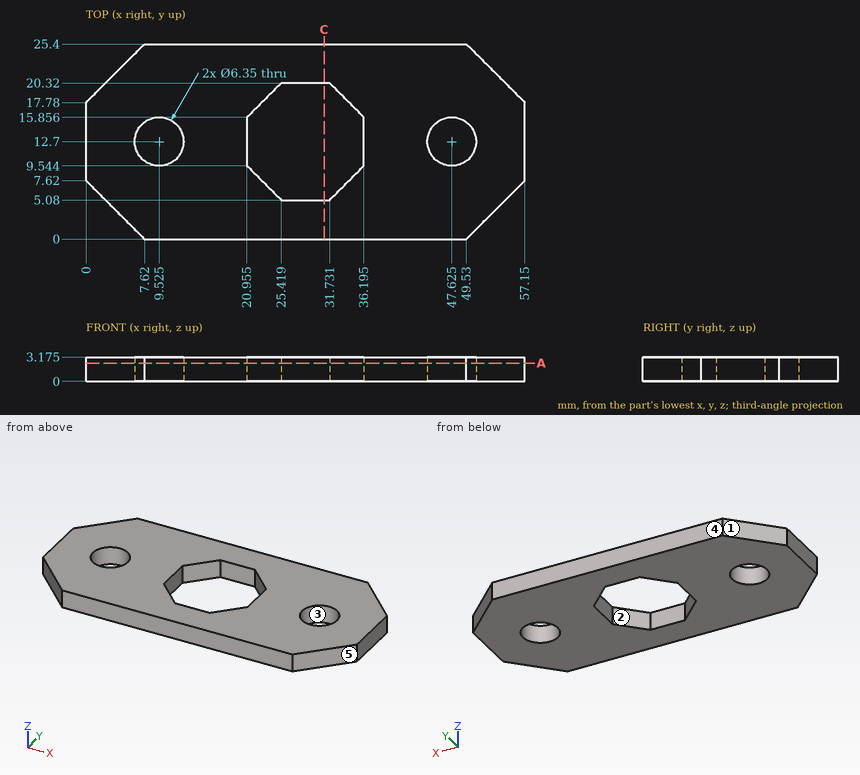
Geometry check sheet. Reference: drawing and pictorial views, mm from the part's lowest x, y, z. A direction names the side the tool comes from. Round coordinates to 2 decimals unless told otherwise and drop trailing zeros. Loops run counter-clockwise (first coordinate to the right, second up) from the corner with the lowest first, then second, coordinate; pieces in that order, holes last. Notation, with made-up numbers: (-12.75, -22) -> (43.25, -22) arc R22 ccw to (43.25, 12) -> close; hole circle Ø10 at (77, 89.5). An arc over 180 degrees is marked (long way). Use a Markdown table: item, result.
(1) Set-up check for the marked faces 1 and 2: record each of +Z, -Z, +X, -X, +Y, -Y from which the full face is reachable in a straight line by a thin tool's end or side.
Calculated:
| item | result |
|---|---|
| face 1 | +Z, -Z, -X, +Y |
| face 2 | +Z, -Z |
(2) Scan lines: probe 1 along Y at (x, z) = (29.5, 2.7); probe 2 along Y at (x, z) = (48, 1.15); probe 3 along X at (y, z) = (7.5, 0.35). Record each from-to range of solid material in increasing order.
Calculated:
| item | result |
|---|---|
| probe 1 | 0 to 5.08, 20.32 to 25.4 |
| probe 2 | 0 to 9.55, 15.85 to 25.4 |
| probe 3 | 0.12 to 23, 34.15 to 57.03 |
(3) Sectioned sample at A-A (z = 2.4). Give the number of separate pieces and of enclosed holes in the cut face, then the cut area to 3 significant figures.
Calculated:
| item | result |
|---|---|
| separate pieces | 1 |
| enclosed holes | 3 |
| area | 1,080 mm² |
(4) Sectioned sample at C-C (x = 31). Enter the section's corners in (y, z) (1 decimal).
Calculated:
| item | result |
|---|---|
| outline | (0, 0) -> (5.1, 0) -> (5.1, 3.2) -> (0, 3.2) -> close; (20.3, 0) -> (25.4, 0) -> (25.4, 3.2) -> (20.3, 3.2) -> close |
(5) Mould release check, pull along Y, two halves, no side actions. Record for the marked faces 3, 4 and 5: released by +Y, released by -Y, zero draft, split by the parting line, or undercut.
Calculated:
| item | result |
|---|---|
| face 3 | undercut |
| face 4 | released by +Y |
| face 5 | released by -Y |
